Part model, mm, in its own coordinate system. Face numbers are marked on the shaded views. Give positions to 0.01 mm unless a question says otherwise; leave off trailing zeros. Write each loop counter-clockwise with the first axis right and the second up, starting at its lowest first coordinate (ties: lowest second). Pieces come first, ordered by that corner, then holes. Notation, with made-up numbers: M 66.5,-27 L 81.5,-27 A12 cw 81.5,-5 Z; hole C 13.5,-18 d10. An arc over 180 degrees is marked long. Use a Markdown table: item, result.
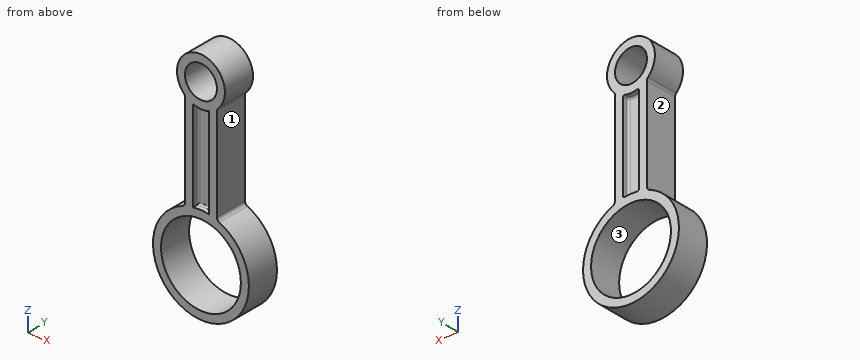
```python
from build123d import *

# Parameters (mm, degrees)
F0_R     = 5.08
F0_R_2   = 12.7
F1_DEPTH = 5.08
F2_R     = 1.27
F4_DEPTH = 1.905
F5_R     = 0.508


# Not quite as in the source:
# - a pattern or mirror of a feature is missing from the dataset's text; its kind, count and spacing are read off the source's solid


with BuildPart() as f1:
    # F0 (on Front) → F1 (new body, symmetric)
    with BuildSketch(Plane.XZ):
        with BuildLine():
            ThreePointArc((5.08, 19.7203873372), (6.9560764803, 22.2891480267), (7.62, 25.4))
            ThreePointArc((7.62, 25.4), (-3.1108519733, 32.3560764803), (-5.08, 19.7203873372))
            ThreePointArc((-5.08, 19.7203873372), (0, 17.78), (5.08, 19.7203873372))
        make_face()
        with Locations((0, 25.4)):
            Circle(F0_R, mode=Mode.SUBTRACT)
        with BuildLine():
            ThreePointArc((5.08, 19.7203873372), (0, 17.78), (-5.08, 19.7203873372))
            Line((-5.08, 19.7203873372), (-5.08, -11.0315902063))
            ThreePointArc((-5.08, -11.0315902063), (0, -10.16), (5.08, -11.0315902063))
            Line((5.08, -11.0315902063), (5.08, 19.7203873372))
        make_face()
        with BuildLine():
            ThreePointArc((5.08, -11.0315902063), (0, -10.16), (-5.08, -11.0315902063))
            ThreePointArc((-5.08, -11.0315902063), (-8.7988181024, -37.8434078933), (15.24, -25.4))
            ThreePointArc((15.24, -25.4), (12.4434078933, -16.6011818976), (5.08, -11.0315902063))
        make_face()
        with Locations((0, -25.4)):
            Circle(F0_R_2, mode=Mode.SUBTRACT)
    extrude(amount=F1_DEPTH, both=True)

    # F2
    f2_edges = [f1.edges().sort_by_distance(p)[0] for p in [
        (-5.08, 0, 19.720387),
        (-5.08, 0, -11.03159),
        (5.08, 0, 19.720387),
        (5.08, 0, -11.03159),
    ]]
    fillet(f2_edges, radius=F2_R)

    # F3 (on face) → F4 (cut)
    with BuildSketch(Plane.XZ.offset(5.08)):
        with BuildLine():
            ThreePointArc((2.54, 18.2157951031), (0, 17.78), (-2.54, 18.2157951031))
            Line((-2.54, 18.2157951031), (-2.54, -10.3731573509))
            ThreePointArc((-2.54, -10.3731573509), (0, -10.16), (2.54, -10.3731573509))
            Line((2.54, -10.3731573509), (2.54, 18.2157951031))
        make_face()
    f4 = extrude(amount=-F4_DEPTH, mode=Mode.SUBTRACT)

    # F4_copies: F4 across plane
    add(f4.mirror(Plane.ZX), mode=Mode.SUBTRACT)

    # F5
    f5_edges = [f1.edges().sort_by_distance(p)[0] for p in [
        (-2.54, -3.175, 3.921319),
        (0, -3.175, 17.78),
        (2.54, -3.175, 3.921319),
        (0, -3.175, -10.16),
        (2.54, 4.1275, -10.373157),
        (2.54, 4.1275, 18.215795),
        (2.54, 3.175, 3.921319),
        (-2.54, 4.1275, 18.215795),
        (0, 3.175, 17.78),
        (-2.54, 4.1275, -10.373157),
        (-2.54, 3.175, 3.921319),
        (0, 3.175, -10.16),
    ]]
    fillet(f5_edges, radius=F5_R)


solid = f1.part
```
1. Cut at C-C, the plane y = 1.5. Give the cut face in (x, z).
Findings below:
| item | result |
|---|---|
| outline | M -5.86,-11.33 A15.24 ccw long 5.86,-11.33 A1.27 cw 5.08,-10.16 L 5.08,19.18 A1.27 cw 5.44,20.07 A7.62 ccw long -5.44,20.07 A1.27 cw -5.08,19.18 L -5.08,-10.16 A1.27 cw Z; hole C 0,-25.4 d25.4; hole C 0,25.4 d10.16 |
2. Cut at B-B, the plane x = 0. Give the cut face in (y, z) (3 decimals).
Findings below:
| item | result |
|---|---|
| outline | M -5.08,-40.64 L 5.08,-40.64 L 5.08,-38.1 L -5.08,-38.1 Z; M -5.08,-12.7 L 5.08,-12.7 L 5.08,-10.16 L 3.683,-10.16 A0.508 cw 3.175,-9.652 L 3.175,17.272 A0.508 cw 3.683,17.78 L 5.08,17.78 L 5.08,20.32 L -5.08,20.32 L -5.08,17.78 L -3.683,17.78 A0.508 cw -3.175,17.272 L -3.175,-9.652 A0.508 cw -3.683,-10.16 L -5.08,-10.16 Z; M -5.08,30.48 L 5.08,30.48 L 5.08,33.02 L -5.08,33.02 Z |
3. Two-plate mould, pull along X, no slides. Class the marked faces 1, 2 and 3: released by +X, released by -X, zero draft, split by the parting line, or undercut.
Findings below:
| item | result |
|---|---|
| face 1 | released by +X |
| face 2 | released by -X |
| face 3 | undercut |
4. Cut at D-D, the plane x = -8.5. Give the cut face in (y, z).
Findings below:
| item | result |
|---|---|
| outline | M -5.08,-38.05 L 5.08,-38.05 L 5.08,-34.84 L -5.08,-34.84 Z; M -5.08,-15.96 L 5.08,-15.96 L 5.08,-12.75 L -5.08,-12.75 Z |
5. Cut at A-A, the plane z = -25.4. Give the cut face in (x, y), then the cut area to 3 significant figures.
Findings below:
| item | result |
|---|---|
| outline | M -15.24,-5.08 L -12.7,-5.08 L -12.7,5.08 L -15.24,5.08 Z; M 12.7,-5.08 L 15.24,-5.08 L 15.24,5.08 L 12.7,5.08 Z |
| area | 51.6 mm2 |
6. Drill centre lines: L1, parallel to Z at x = 0, y = -2.5; L2, parallel to Z at x = 6, y = 3; L3, parallel to X at y = 4.5, z = 5.5. Where is each one in solid material? Low to high.
Findings below:
| item | result |
|---|---|
| L1 | -40.64 to -38.1, -12.7 to 20.32, 30.48 to 33.02 |
| L2 | -39.41 to -36.59, -14.21 to -11.39, 20.7 to 30.1 |
| L3 | -5.08 to -2.54, 2.54 to 5.08 |
7. Drop flat-ended pins along their axis: P1, Ø1.5, axis at y = -1, z = 15, coming from the -X side; P2, Ø4.5, axis at x = 0.5, z = -1.5, coming from the -Y side; P3, Ø4, axis at x = -3, y = -1.5, coming from the -Z side; P4, Ø9, axis at x = 0, z = 25.4, coming from the -Y side. Give the stop position or say it passes through.
Findings below:
| item | result |
|---|---|
| P1 | x = -5.08 |
| P2 | y = -5.08 |
| P3 | z = -40.61 |
| P4 | through |
